```python
from build123d import *

# Parameters (mm, degrees)
F1_DEPTH = 15


with BuildPart() as f1:
    # F0 (on Front) → F1 (new body)
    with BuildSketch(Plane.XZ):
        with BuildLine():
            Line((24, 0), (0, 0))
            Line((0, 0), (0, -2))
            Line((0, -2), (26, -2))
            ThreePointArc((26, -2), (26.707107, -1.707107), (27, -1))
            Line((27, -1), (27, 0))
            Line((27, 0), (27, 15))
            Line((27, 15), (25, 15))
            Line((25, 15), (25, 1))
            ThreePointArc((25, 1), (24.707107, 0.292893), (24, 0))
        make_face()
    extrude(amount=F1_DEPTH)


solid = f1.part
```
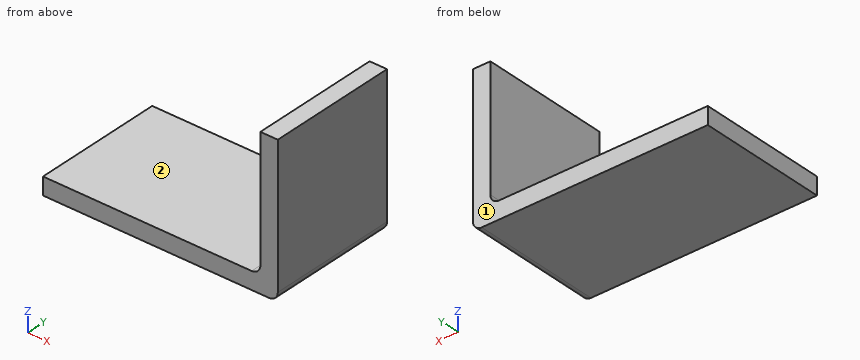
The listing builds one solid part. Answer for the finished solid, in the listing's coordinates (mm). Face numbers are marked on the shaded views. A direction names the side the tool comes from. Round coordinates to 2 decimals unless told otherwise and drop trailing zeros. Order: outer loops, then holes, each group sorted by start corner. A loop starts at its lowest first (then second) coordinate and runs counter-clockwise, first axis right, second up. Notation, with made-up numbers: (-33.5, 16.5) -> (-21.5, 16.5) arc R20 cw to (-21.5, 55.5) -> close; hole circle Ø11 at (-7, 22.5). An arc over 180 degrees is marked (long way). Answer as CSV lines item,"result".
Q1. A cutting plane is placed at C-C on x = 10.75. Determine the outline of the cut face in (y, z).
Computed values:
outline,"(-15, -2) -> (0, -2) -> (0, 0) -> (-15, 0) -> close"
Q2. A cutting plane is placed at A-A on y = -5. Determine the outline of the cut face in (x, z).
Computed values:
outline,"(0, -2) -> (26, -2) arc R1 ccw to (27, -1) -> (27, 15) -> (25, 15) -> (25, 1) arc R1 cw to (24, 0) -> (0, 0) -> close"
Q3. Given pin 1 (5 mm diameter, centred on y = -7, z = 1, fed in from -X); pin 2 (1.5 mm diameter, centred on y = -13, z = 6.5, fed in from -X); pin 3 (4.5 mm diameter, centred on x = 9, y = -7.5, fed in from +Z), each flat-ended and moving along its own axis, determine where each tip first touches the part or whether it passes through.
Computed values:
pin 1,"stops at x = 0"
pin 2,"stops at x = 25"
pin 3,"stops at z = 0"
Q4. Which of the six approach directions +Z, -Z, +X, -X, +Y, -Y give full straight-line access (tool end or side, diameter ignored) to the marked faces 1 and 2?
Computed values:
face 1,"+Z, -Z, +X, -X, +Y"
face 2,"+Z, -X, +Y, -Y"
Q5. Consider line 1 (X direction, y = -3, z = 4.25); line 2 (Z direction, x = 7.5, y = -9.75); line 3 (Z direction, x = 26.25, y = -5.75). Determine where each line is inside the solid, lowest interval first. Write a range as from..to.
Computed values:
line 1,"x = 25..27"
line 2,"z = -2..0"
line 3,"z = -1.97..15"
Q6. A cutting plane is placed at B-B on z = 4.5. Determine the outline of the cut face in (x, y), plus the area to 3 significant figures.
Computed values:
outline,"(25, -15) -> (27, -15) -> (27, 0) -> (25, 0) -> close"
area,"30.0 mm^2"
